from build123d import *

# Parameters (mm, degrees)
BOSS_EXTRU_1_DEPTH = 75


with BuildPart() as part:
    # Esquisse1 → Boss.-Extru.1 (new body)
    with BuildSketch(Plane(origin=(0, 0, 0), x_dir=(0, 0, -1), z_dir=(1, 0, 0))):
        with BuildLine():
            Line((1.448022121, -1.379576725), (1.448022121, 1.379576723))
            ThreePointArc((1.448022121, 1.379576723), (1, 1.732050807), (0.470737428, 1.943812304))
            Line((0.470737428, 1.943812304), (-1.918759551, 0.56423558))
            ThreePointArc((-1.918759551, 0.56423558), (-1.979585702, 0.285027104), (-2, 0))
            ThreePointArc((-2, 0), (-1.979585702, -0.285027104), (-1.918759551, -0.564235579))
            Line((-1.918759551, -0.564235579), (0.470737429, -1.943812304))
            ThreePointArc((0.470737429, -1.943812304), (1, -1.732050808), (1.448022121, -1.379576725))
        make_face()
    extrude(amount=BOSS_EXTRU_1_DEPTH)


solid = part.part
Geometry check sheet. Reference: the model listing, model coordinates, mm. Coordinates: 2 decimals unless noted, no trailing zeros. Order: outer loops, then holes, each group sorted by start corner. A loop starts at its lowest first (then second) coordinate and runs counter-clockwise, first axis right, second up. Notation, with made-up numbers: M 51,-29 L 94,-29 A18 ccw 94,6 Z; hole C -3.5,-5 d9. An arc over 180 degrees is marked long. Use CSV: the item, a comma, the result in double quotes.
Item 1: Thickness scan on line 1 along Z through (x, y) = (72, 0.2); line 2 along Y through (x, z) = (24.5, -0.5); line 3 along Z through (x, y) = (20.5, -0.5). Record the ranges inside material, lowest first.
Returned:
line 1,"z = -1.45 to 1.99"
line 2,"y = -1.94 to 1.94"
line 3,"z = -1.45 to 1.94"
Item 2: Cross-section at A-A on x = 5. Record the cut outline in (y, z), then the cut area to 4 significant figures.
Returned:
outline,"M -1.94,-0.47 A2 ccw -1.38,-1.45 L 1.38,-1.45 A2 ccw 1.94,-0.47 L 0.56,1.92 A2 ccw -0.56,1.92 Z"
area,"9.425 mm2"
Item 3: Cross-section at B-B on z = 0.5. Record the cut outline in (x, y), then the cut area to 3 significant figures.
Returned:
outline,"M 0,-1.38 L 75,-1.38 L 75,1.38 L 0,1.38 Z"
area,"208 mm2"
